Could you check a few things on this model? Use its own coordinates, in mm. A direction names the side the tool comes from. Coordinates: 2 decimals unless noted, no trailing zeros. Loops run counter-clockwise (first coordinate to the right, second up) from the corner with the lowest first, then second, coordinate; pieces in that order, holes last. Notation, with made-up numbers: (4, 49) - (58, 49) arc R13 cw to (58, 61) - close; hole circle Ø2 at (26, 46.25). An arc over 180 degrees is marked (long way). Put each result on its own line as item: value. Start each with the question number.
```python
from build123d import *

# Parameters (mm, degrees)
BOSS_EXTRUDE1_DEPTH = 25
CUT_EXTRUDE2_DEPTH  = 4
FILLET6_R           = 10
FILLET7_R           = 5
BOSS_EXTRUDE2_DEPTH = 20
SKETCH8_R           = 1.6
CUT_EXTRUDE3_DEPTH  = 2
BOSS_EXTRUDE3_DEPTH = 14
SKETCH11_R          = 1.6
CUT_EXTRUDE4_DEPTH  = 2


with BuildPart() as part:
    # Sketch1 → Boss-Extrude1 (new body)
    with BuildSketch(Plane(origin=(0, 0, 0), x_dir=(0, 0, -1), z_dir=(1, 0, 0))):
        Polygon((0, 0), (-130, 0), (-130, 5), (-100.000366453, 5.148280317), (-91.235719846, 14), (114, 14), (114, 0), (74, 0), (74, 4.5), (0, 4.5), align=None)
    extrude(amount=BOSS_EXTRUDE1_DEPTH)

    # Sketch6 → Cut-Extrude2 (cut)
    with BuildSketch(Plane(origin=(25, 0, 0), x_dir=(0, 0, -1), z_dir=(1, 0, 0))):
        Polygon((-100.876178749, 0), (114, 0), (114, 11), (-89.984384146, 11), align=None)
    cut_extrude2 = extrude(amount=-CUT_EXTRUDE2_DEPTH, mode=Mode.SUBTRACT)

    # Mirror3: Cut-Extrude2 across plane
    add(cut_extrude2.mirror(Plane(origin=(12.5, 0, 0), x_dir=(0, 0, 1), z_dir=(1, 0, 0))), mode=Mode.SUBTRACT)

    # Fillet6
    fillet6_edges = [part.edges().sort_by_distance(p)[0] for p in [
        (23, 0, 100.876178749),
        (23, 11, 89.984384146),
        (2, 0, 100.876178749),
        (2, 11, 89.984384146),
    ]]
    fillet(fillet6_edges, radius=FILLET6_R)

    # Fillet7
    fillet7_edges = [part.edges().sort_by_distance(p)[0] for p in [
        (12.5, 5.148280317, 100.000366453),
        (12.5, 14, 91.235719846),
    ]]
    fillet(fillet7_edges, radius=FILLET7_R)

    # Sketch7 → Boss-Extrude2 (add)
    with BuildSketch(Plane.XZ):
        Polygon((21, 85), (4, 85), (4, 64), (6, 64), (6, 83), (19, 83), (19, 64), (21, 64), align=None)
    extrude(amount=BOSS_EXTRUDE2_DEPTH)

    # Sketch8 → Cut-Extrude3 (cut)
    with BuildSketch(Plane.XY.offset(85)):
        with Locations((15.75, -16.25)):
            Circle(SKETCH8_R)
        with Locations((9.25, -16.25)):
            Circle(SKETCH8_R)
        with Locations((9.25, -8.75)):
            Circle(SKETCH8_R)
        with Locations((15.75, -8.75)):
            Circle(SKETCH8_R)
    extrude(amount=-CUT_EXTRUDE3_DEPTH, mode=Mode.SUBTRACT)

    # Sketch9 → Boss-Extrude3 (add)
    with BuildSketch(Plane.XZ):
        Polygon((4, -114), (21, -114), (21, -93), (19, -93), (19, -112), (6, -112), (6, -93), (4, -93), align=None)
    extrude(amount=BOSS_EXTRUDE3_DEPTH)

    # Sketch11 → Cut-Extrude4 (cut)
    with BuildSketch(Plane(origin=(0, 0, -114), x_dir=(-1, 0, 0), z_dir=(0, 0, -1))):
        with Locations((-9.25, -10.25)):
            Circle(SKETCH11_R)
        with Locations((-15.75, -10.25)):
            Circle(SKETCH11_R)
    extrude(amount=-CUT_EXTRUDE4_DEPTH, mode=Mode.SUBTRACT)


solid = part.part
```
(1) I want a section at B-B on z = -85.5. List the corners of the cut face in (x, y) for me.
(2) For pin 1 Ø10 at (x, z) = (12.5, -67.5) entering from -Y; pin 2 Ø15.5 at (y, z) = (-7.5, -98.5) entering from +X; pin 3 Ø12 at (x, z) = (9, 101) entering from -Y, each with a flat end and sliding along its axis, tell me the tip position at first contact or that it passes through.
(3) If we mould it in two halves opening along X, with no side actions, what happens to faces 1 (the flat face through (6, -10, 73)), 2 (the cylindrical face through (2.03, 0.75, 101.25)), 3 (the flat face through (21, 6, -6)), 4 (the flat face through (19, -7, -102))? For each: pulls with the +X half, pulls with the -X half, needs draft (parallel to the pull), parting line crosses it, or undercut.
(4) I need wall thicknesses on L1, parallel to Y at x = 15.75, z = 83.5; L2, parallel to Z at x = 20, y = -12; L3, parallel to X at y = -8, z = 84. Which ranges of each line are inside material? Lowest first, please. Write a range as [from, to].
(5) Which directions (+Z, -Z, +X, -X, +Y, -Y) give clear straight access to the entire face, cutting with the end or side of a thin tool? Please do faces 5 (the flat face through (13, -7, -112)), 6 (the flat face through (2, 11, -15)), 7 (the flat face through (12, 2, 0)), 8 (the flat face through (13, -10, 85)).
(6) I want a section at A-A on y = -4. List the corners of the cut face in (x, z) for me.
Answer sheet:
1. outline: (0, 11) - (4, 11) - (4, 0) - (21, 0) - (21, 11) - (25, 11) - (25, 14) - (0, 14) - close
2. pin 1: stops at y = 4.5
2. pin 2: stops at x = 21
2. pin 3: stops at y = 0
3. face 1: undercut
3. face 2: needs draft
3. face 3: pulls with the +X half
3. face 4: undercut
4. L1: y = [-20, -17.85], [-14.65, -10.35], [-7.15, 14]
4. L2: z = [-114, -93], [64, 85]
4. L3: x = [4, 7.84], [10.66, 14.34], [17.16, 21]
5. face 5: -Y
5. face 6: -Z, -X, -Y
5. face 7: +X, -X, -Y
5. face 8: +Z, +X, -X, -Y
6. outline: (4, -114) - (21, -114) - (21, -93) - (19, -93) - (19, -112) - (6, -112) - (6, -93) - (4, -93) - close; (4, 64) - (6, 64) - (6, 83) - (19, 83) - (19, 64) - (21, 64) - (21, 85) - (4, 85) - close
